```python
from build123d import *

# Parameters (mm, degrees)
F0_R         = 11.1125
F1_DEPTH     = 3.048
F0_R_2       = 1.905
F2_DEPTH     = 1.524
F3_R         = 1.1286206983
F4_T6_ANGLE  = 269.6278921261
F4_S7_R      = 3.429
F4_T8_DEPTH  = 22
F4_T12_ANGLE = 89.6035333551
F4_S13_R     = 3.429
F4_T14_DEPTH = 11


# Not quite as in the source:
# - a fillet or chamfer that OpenCascade refuses, or shapes differently, is made with other operations: its cross-section is extruded or revolved along the edge and cut away or added


with BuildPart() as f1:
    # F0 (on Front) → F1 (new body)
    with BuildSketch(Plane.XZ):
        with BuildLine():
            ThreePointArc((-2.05101646, 14.0111773856), (-9.2594908518, -10.713617009), (14.1605, 0))
            ThreePointArc((14.1605, 0), (10.713617009, 9.2594908518), (2.05101646, 14.0111773856))
            ThreePointArc((2.05101646, 14.0111773856), (0, 13.3301534555), (-2.05101646, 14.0111773856))
        make_face()
        Circle(F0_R, mode=Mode.SUBTRACT)
        with BuildLine():
            ThreePointArc((-2.05101646, 14.0111773856), (0, 13.3301534555), (2.05101646, 14.0111773856))
            ThreePointArc((2.05101646, 14.0111773856), (0, 14.1605), (-2.05101646, 14.0111773856))
        make_face()
    extrude(amount=F1_DEPTH)

    # F0 (on Front) → F2 (join)
    with BuildSketch(Plane.XZ):
        with BuildLine():
            ThreePointArc((-2.05101646, 14.0111773856), (0, 14.1605), (2.05101646, 14.0111773856))
            ThreePointArc((2.05101646, 14.0111773856), (3.065206065, 15.2220936716), (3.429, 16.7591534555))
            ThreePointArc((3.429, 16.7591534555), (-1.5370597839, 19.8243595205), (-2.05101646, 14.0111773856))
        make_face()
        with Locations((0, 16.7591534555)):
            Circle(F0_R_2, mode=Mode.SUBTRACT)
    extrude(amount=F2_DEPTH)

    # F3
    f3_edges = [f1.edges().sort_by_distance(p)[0] for p in [
        (11.1125, -1.524, 0),
        (-11.1125, 0, 0),
        (-11.1125, -3.048, 0),
    ]]
    fillet(f3_edges, radius=F3_R)

    # F4: chamfer of 0.762 on 2 edges, made by hand

    # F4_s1 → F4_t2 (revolve, cut)
    with BuildSketch(Plane.XY):
        Polygon((14.1605, -2.286), (13.3985, -3.048), (14.1605, -3.048), align=None)
    revolve(axis=Axis((0, -3.048, 0), (0, -1, 0)), mode=Mode.SUBTRACT)


with BuildPart() as f4_tool4:
    # F4_s5 → F4_t6 (revolve)
    with BuildSketch(Plane(origin=(0, 0, 0), x_dir=(0, 1, 0), z_dir=(0.9999789108, 0, 0.0064944619))):
        Polygon((0, 13.3985), (-0.762, 14.1605), (0, 14.1605), align=None)
    revolve(axis=Axis((0, 0, 0), (0, -1, 0)), revolution_arc=F4_T6_ANGLE)

    # F4_s7 → F4_t8 (cut, symmetric)
    with BuildSketch(Plane.XZ.offset(0.4)):
        with Locations((0, 16.7591534555)):
            Circle(F4_S7_R)
    extrude(amount=F4_T8_DEPTH, both=True, mode=Mode.SUBTRACT)


with BuildPart() as f1_1:
    add(f1.part)

    # F4_t3: cut F4_tool4
    add(f4_tool4.part, mode=Mode.SUBTRACT)


with BuildPart() as f4_tool10:
    # F4_s11 → F4_t12 (revolve)
    with BuildSketch(Plane.XY):
        Polygon((13.3985, 0), (14.1605, -0.762), (14.1605, 0), align=None)
    revolve(axis=Axis((0, 0, 0), (0, -1, 0)), revolution_arc=F4_T12_ANGLE)

    # F4_s13 → F4_t14 (cut, symmetric)
    with BuildSketch(Plane.XZ.offset(0.4)):
        with Locations((0, 16.7591534555)):
            Circle(F4_S13_R)
    extrude(amount=F4_T14_DEPTH, both=True, mode=Mode.SUBTRACT)


with BuildPart() as f1_2:
    add(f1_1.part)

    # F4_t9: cut F4_tool10
    add(f4_tool10.part, mode=Mode.SUBTRACT)


solid = f1_2.part
```
Source: CAD feature listing. Evaluate the final solid. Frame: model axes, mm. Give positions to 0.01 mm unless a question says otherwise; leave off trailing zeros. Loops run counter-clockwise (first coordinate to the right, second up) from the corner with the lowest first, then second, coordinate; pieces in that order, holes last. Notation, with made-up numbers: M 78,21 L 110,21 A7 cw 110,29 Z; hole C 1.5,66 d5. An arc over 180 degrees is marked long. Put each result on its own line as item: value.
Q1. Section A-A (x = 0). Return the cut outline in (y, z), and give its area (3 significant figures).
Response values:
outline: M -3.05,-13.4 L -2.29,-14.16 L -0.76,-14.16 L 0,-13.4 L 0,-12.24 A1.13 ccw -1.13,-11.11 L -1.92,-11.11 A1.13 ccw -3.05,-12.24 Z; M -3.05,12.24 A1.13 ccw -1.92,11.11 L -1.13,11.11 A1.13 ccw 0,12.24 L 0,14.85 L -1.52,14.85 L -1.52,14.16 L -2.29,14.16 L -3.05,13.4 Z; M -1.52,18.66 L 0,18.66 L 0,20.19 L -1.52,20.19 Z
area: 20.0 mm²
Q2. Pin query (flat end, axial travel): P1, Ø1.5, axis at y = -1.5, z = -4, coming from the -X side; P2, Ø1.9, axis at x = 0, z = 18.5, coming from the -Y side. Return the tip coordinate at first contact, or that it passes through.
Response values:
P1: stops at x = -13.78
P2: stops at y = -1.52
Q3. Mould query, pull axis Z, two halves, no side actions, for faces 1 (the cylindrical face through (-0.248, -0.751, 18.648)), 2 (the flat face through (-1, -1.524, 19)). Classes: released by +Z, released by -Z, zero draft, split by the parting line, or undercut.
Response values:
face 1: undercut
face 2: zero draft
Q4. Line query: probe 1 along Z at (x, y) = (0, -1.1); probe 2 along Z at (x, y) = (0, -0.45); probe 3 along Z at (x, y) = (0, -1.6). Output: solid intervals per line, ascending. Write a range as [from, to].
Response values:
probe 1: z = [-14.16, -11.11], [11.11, 14.85], [18.66, 20.19]
probe 2: z = [-13.85, -11.34], [11.34, 14.85], [18.66, 20.19]
probe 3: z = [-14.16, -11.11], [11.11, 14.16]
Q5. Section B-B (y = -0.4). Return the cut outline in (x, z) (1 decimal).
Response values:
outline: M -1.6,13.7 A13.8 ccw long 1.6,13.7 A3.4 ccw long Z; hole C 0,0 d22.8; hole C 0,16.8 d3.8
Q6. Section C-C (x = -3). Count the separate pieces of the cut face and the enclosed holes in it, and give its area (3 significant figures).
Response values:
separate pieces: 3
enclosed holes: 0
area: 21.9 mm²
